Source: CAD feature listing. Evaluate the final solid. Frame: model axes, mm. A direction names the side the tool comes from. Round coordinates to 2 decimals unless told otherwise and drop trailing zeros. Loops run counter-clockwise (first coordinate to the right, second up) from the corner with the lowest first, then second, coordinate; pieces in that order, holes last. Notation, with made-up numbers: M 9,62.5 L 24,62.5 A7 ccw 24,69.5 Z; hole C -2.75,-11 d8. An arc over 180 degrees is marked long. Write each question's results on one line, items separated by ' | '. Start each with the question number.
1. Set-up query: faces 5 (the cylindrical face through (50.492, 48.304, 26.451)), 6 (the cylindrical face through (26, 10, 5)), 7 (the flat face through (80, 44, 15)). Return all of +Z, -Z, +X, -X, +Y, -Y with unobstructed straight access to the full face (end or side cutting, diameter ignored); none if empty.
2. Draft query along X for faces 1 (the flat face through (0, 44, 15)), 2 (the flat face through (41, 0, 15)), 3 (the cylindrical face through (66.846, 76.451, 5.07)), 4 (the cylindrical face through (26.59, 65.04, 3.55)). Return one class per face: released by +X, released by -X, zero draft, split by the parting line, or undercut.
3. Section A-A on y = 45. Output: boundary loops of the cut face in (x, z).
4. Contact query for flat-ended pins moving along their axis: pin 1 Ø7 at (x, y) = (30, 10) entering from -Z; pin 2 Ø5 at (x, y) = (30, 80) entering from -Z; pin 3 Ø1.5 at (x, y) = (26.75, 63.8) entering from -Z. Output: stop coordinate, or through.
5. Ray query, line 1 (X direction, y = 10, z = 4.5); line 2 (Y direction, x = 65, z = 6.5); line 3 (Y direction, x = 53.25, z = 3.25). Return the intervals inside material, ascending.
6. Section D-D on z = 5.25. Output: boundary loops of the cut face in (x, y).
7. Section C-C on z = 21.5. Output: boundary loops of the cut face in (x, y).
8. Section B-B on x = 40. Output: boundary loops of the cut face in (y, z), and give its area (3 significant figures).
from build123d import *

# Parameters (mm, degrees)
SKETCH1_W                      = 80
SKETCH1_H                      = 90
BOSS_EXTRUDE1_DEPTH            = 30
F_2_5_2_5_DIAMETER_HOLE1_D     = 2.5
F_2_5_2_5_DIAMETER_HOLE1_DEPTH = 7
F_2_5_2_5_DIAMETER_HOLE1_TIP   = 0.721687836
F_8_0_8_DIAMETER_HOLE1_D       = 8
F_8_0_8_DIAMETER_HOLE1_DEPTH   = 10
F_8_0_8_DIAMETER_HOLE1_TIP     = 2.309401077


with BuildPart() as part:
    # Sketch1 → Boss-Extrude1 (new body)
    with BuildSketch(Plane(origin=(0, 0, 0), x_dir=(-1, 0, 0), z_dir=(0, 0, -1))):
        with Locations((-40, 45)):
            Rectangle(SKETCH1_W, SKETCH1_H)
    extrude(amount=-BOSS_EXTRUDE1_DEPTH)

    # Sketch2 → Cut-Revolve1 (revolve, cut)
    with BuildSketch(Plane(origin=(0, 45, 0), x_dir=(-1, 0, 0), z_dir=(0, -1, 0)), mode=Mode.PRIVATE) as cut_revolve1_sk:
        Polygon((-29, 0), (-40, 0), (-40, -30), (-29, -30), (-29, -23), (-30, -23), (-30, -8), (-29, -8), align=None)
    revolve(cut_revolve1_sk.sketch.rotate(Axis((40, 45, 0), (0, 0, 1)), 180), axis=Axis((40, 45, 0), (0, 0, 1)), mode=Mode.SUBTRACT)

    # Ø2.5 (2.5) Diameter Hole1
    with Locations(Plane(origin=(0, 0, 0), x_dir=(-1, 0, 0), z_dir=(0, 0, -1))):
        with Locations((-26.75, 63.799933511), (-53.25, 26.200066489)):
            Hole(F_2_5_2_5_DIAMETER_HOLE1_D / 2, depth=F_2_5_2_5_DIAMETER_HOLE1_DEPTH)
            with Locations((0, 0, -(F_2_5_2_5_DIAMETER_HOLE1_DEPTH + F_2_5_2_5_DIAMETER_HOLE1_TIP / 2))):  # 120° drill point
                Cone(0, F_2_5_2_5_DIAMETER_HOLE1_D / 2, F_2_5_2_5_DIAMETER_HOLE1_TIP, mode=Mode.SUBTRACT)

    # Ø8.0 (8) Diameter Hole1
    with Locations(Plane(origin=(0, 0, 0), x_dir=(-1, 0, 0), z_dir=(0, 0, -1))):
        with Locations((-30, 10), (-30, 80), (-65, 10), (-65, 80)):
            Hole(F_8_0_8_DIAMETER_HOLE1_D / 2, depth=F_8_0_8_DIAMETER_HOLE1_DEPTH)
            with Locations((0, 0, -(F_8_0_8_DIAMETER_HOLE1_DEPTH + F_8_0_8_DIAMETER_HOLE1_TIP / 2))):  # 120° drill point
                Cone(0, F_8_0_8_DIAMETER_HOLE1_D / 2, F_8_0_8_DIAMETER_HOLE1_TIP, mode=Mode.SUBTRACT)


solid = part.part
Taken from the geometry:
1) face 5: +Z | face 6: -Z | face 7: +Z, -Z, +X, +Y, -Y
2) face 1: released by -X | face 2: zero draft | face 3: undercut | face 4: undercut
3) outline: M 0,0 L 29,0 L 29,8 L 30,8 L 30,23 L 29,23 L 29,30 L 0,30 Z; M 50,8 L 51,8 L 51,0 L 80,0 L 80,30 L 51,30 L 51,23 L 50,23 Z
4) pin 1: z = 10.29 | pin 2: z = 10.87 | pin 3: z = 7.29
5) line 1: 0 to 26, 34 to 61, 69 to 80 | line 2: 0 to 6, 14 to 76, 84 to 90 | line 3: 0 to 24.95, 27.45 to 90
6) outline: M 0,0 L 80,0 L 80,90 L 0,90 Z; hole C 26.75,63.8 d2.5; hole C 30,10 d8; hole C 30,80 d8; hole C 40,45 d22; hole C 53.25,26.2 d2.5; hole C 65,10 d8; hole C 65,80 d8
7) outline: M 0,0 L 80,0 L 80,90 L 0,90 Z; hole C 40,45 d20
8) outline: M 0,0 L 34,0 L 34,8 L 35,8 L 35,23 L 34,23 L 34,30 L 0,30 Z; M 55,8 L 56,8 L 56,0 L 90,0 L 90,30 L 56,30 L 56,23 L 55,23 Z | area: 2,070 mm^2
